```python
from build123d import *

# Parameters (mm, degrees)
BASEHEAD_DEPTH     = 10.75
THDSCHPAT_COUNT    = 18
THDSCHPAT_PITCH    = 1.944444444
SKETCH4_R          = 4.25
CUT_EXTRUDE1_DEPTH = 56.75


with BuildPart() as part:
    # Sketch1 → BaseHead (new body)
    with BuildSketch(Plane(origin=(0, 0, 0), x_dir=(0, 0, -1), z_dir=(1, 0, 0))):
        Polygon((12, 6.92820323), (12, -6.92820323), (0, -13.856406461), (-12, -6.92820323), (-12, 6.92820323), (0, 13.856406461), align=None)
    extrude(amount=BASEHEAD_DEPTH)

    # BodySke → BaseBody (revolve)
    with BuildSketch(Plane.XY):
        Polygon((0, 0), (55.75, 0), (55.75, 6.8985), (54.6485, 8), (0, 8), align=None)
    revolve(axis=Axis((0, 0, 0), (1, 0, 0)))

    # Sketch3 → HeadChamfer (revolve, cut)
    with BuildSketch(Plane.XY):
        Polygon((0, 12), (3.958548116, 18.856406461), (3.958548116, 23.856406461), (-10, 23.856406461), (-10, 12), align=None)
    revolve(axis=Axis((0, 0, 0), (1, 0, 0)), mode=Mode.SUBTRACT)

    # ThdSchSke → ThreadSchematic (revolve, cut)
    with BuildSketch(Plane.XY):
        Polygon((20.75, -6.8985), (19.978721397, -8), (19.978721397, -10), (21.521278603, -10), (21.521278603, -8), align=None)
    threadschematic = revolve(axis=Axis((-3.175, 0, 0), (1, 0, 0)), mode=Mode.SUBTRACT)

    # ThdSchPat: ThreadSchematic ×18
    with Locations(*[(i * THDSCHPAT_PITCH, 0, 0) for i in range(1, THDSCHPAT_COUNT)]):
        add(threadschematic, mode=Mode.SUBTRACT)

    # Sketch4 → Cut-Extrude1 (cut, through all)
    with BuildSketch(Plane.ZY):
        Circle(SKETCH4_R)
    extrude(amount=-CUT_EXTRUDE1_DEPTH, mode=Mode.SUBTRACT)


solid = part.part
```
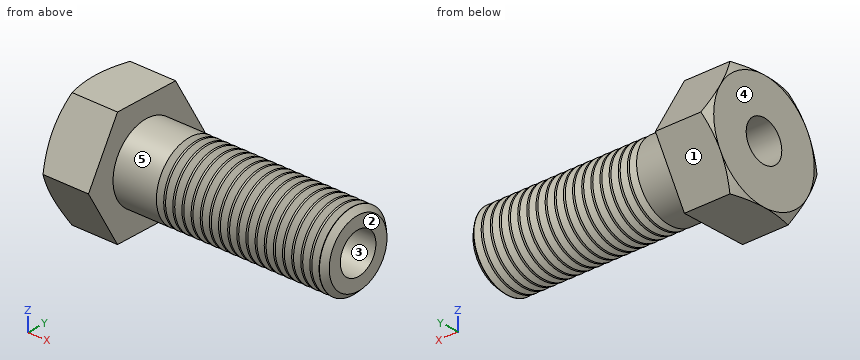
Could you check a few things on this model? Use its own coordinates, in mm. Face numbers are marked on the shaded views. A direction names the side the tool comes from. Round coordinates to 2 decimals unless told otherwise and drop trailing zeros. Loops run counter-clockwise (first coordinate to the right, second up) from the corner with the lowest first, then second, coordinate; pieces in that order, holes last. Notation, with made-up numbers: (61, 3.25) - (98, 3.25) arc R14 cw to (98, 22.25) - close; hole circle Ø4 at (-31.5, 2). An arc over 180 degrees is marked (long way). Answer in a Markdown table with one row per item. Add a question column.
(1) I'm going to push flat-ended pins straight in: pin 1 (13.5 mm diameter, centred on y = 0, z = 0, fed in from +X); pin 2 (2 mm diameter, centred on x = 34.5, y = 7, fed in from +Z); pin 3 (10 mm diameter, centred on x = 30.5, y = 5.5, fed in from +Z); pin 4 (5 mm diameter, centred on x = 46, z = -6, fed in from +Y). Where does each tip first touch, or does it pass through?
(2) If we mould it in two halves opening along Y, with no side actions, what happens to the marked faces 1, 2 and 3? For each: pulls with the +Y half, pulls with the -Y half, needs draft (parallel to the pull), parting line crosses it, or undercut.
(3) If we section it at A-A (x = 10): Please give me the cut outline in (y, z), plus the area to 3 significant figures.
(4) For the marked faces 4 and 5, which set-ups out of +Z, -Z, +X, -X, +Y, -Y let a thin tool reach every point of the face, with its end or its side?
(5) I need wall thicknesses on line 1 along Y through (x, z) = (15, 0); line 2 along X through (y, z) = (-7.75, -5.25); line 3 along Z through (x, y) = (10, -2.25). Which ranges of each line are inside material? Lowest first, please.
Model answer:
| question | item | result |
|---|---|---|
| 1 | pin 1 | stops at x = 55.75 |
| 1 | pin 2 | stops at z = 5.02 |
| 1 | pin 3 | stops at z = 7.98 |
| 1 | pin 4 | stops at y = 7.14 |
| 2 | face 1 | pulls with the +Y half |
| 2 | face 2 | needs draft |
| 2 | face 3 | undercut |
| 3 | outline | (-13.86, 0) - (-6.93, -12) - (6.93, -12) - (13.86, 0) - (6.93, 12) - (-6.93, 12) - close; hole circle Ø8.5 at (0, 0) |
| 3 | area | 442 mm² |
| 4 | face 4 | +Z, -Z, -X, +Y, -Y |
| 4 | face 5 | +X |
| 5 | line 1 | y = -8 to -4.25, 4.25 to 8 |
| 5 | line 2 | x = 0 to 10.75 |
| 5 | line 3 | z = -12 to -3.61, 3.61 to 12 |
